Work out the finished part from the listing and answer in its coordinate system (mm). Face numbers are marked on the shaded views. A direction names the side the tool comes from. Round coordinates to 2 decimals unless told otherwise and drop trailing zeros. Order: outer loops, then holes, each group sorted by start corner. A loop starts at its lowest first (then second) coordinate and runs counter-clockwise, first axis right, second up. Notation, with made-up numbers: (-12, 83.5) - (31, 83.5) arc R27 cw to (31, 119.5) - close; hole circle Ø5 at (20, -11.75). An arc over 180 degrees is marked (long way). Put each result on its own line as item: value.
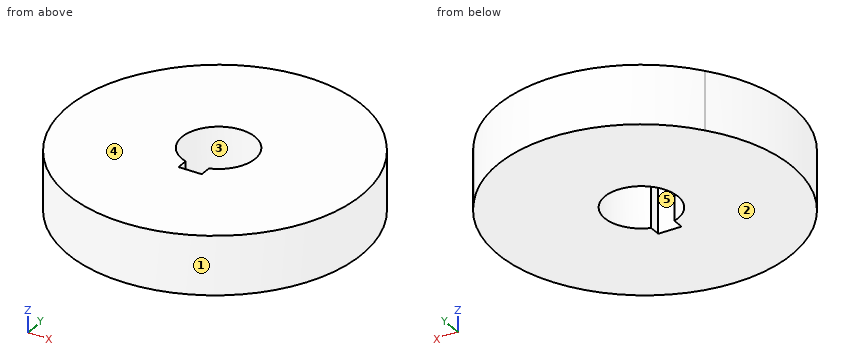
```python
from build123d import *

# Parameters (mm, degrees)
F1_DEPTH = 200
F3_DEPTH = 469.9


# Not quite as in the source:
# - a feature names something its author has since deleted; it is built from what else it names


with BuildPart() as f1:
    # F0 (on Top) → F1 (new body)
    with BuildSketch(Plane.XY):
        with BuildLine():
            ThreePointArc((-396.7193466419, 287.6), (-151.1746012819, -466.0968138995), (490, 0))
            ThreePointArc((490, 0), (466.0968138995, 151.1746012818), (396.7193466419, 287.6))
            ThreePointArc((396.7193466419, 287.6), (0, 482), (-396.7193466419, 287.6))
        make_face()
        with BuildLine():
            ThreePointArc((396.7193466419, 287.6), (466.0968138995, 151.1746012818), (490, 0))
            ThreePointArc((490, 0), (-151.1746012819, -466.0968138995), (-396.7193466419, 287.6))
            ThreePointArc((-396.7193466419, 287.6), (-162.5590477115, -494.9511090703), (502, -20))
            ThreePointArc((502, -20), (474.9511090703, 142.5590477115), (396.7193466419, 287.6))
        make_face()
        with BuildLine():
            ThreePointArc((-396.7193466419, 287.6), (0, 482), (396.7193466419, 287.6))
            ThreePointArc((396.7193466419, 287.6), (0, 490), (-396.7193466419, 287.6))
        make_face()
    extrude(amount=-F1_DEPTH)

    # F2 (on Top) → F3 (cut)
    with BuildSketch(Plane.XY):
        with BuildLine():
            ThreePointArc((40, -118.4271928233), (101.5504800579, -72.8868986856), (125, 0))
            ThreePointArc((125, 0), (-72.8868986856, 101.5504800579), (-40, -118.4271928233))
            Line((-40, -118.4271928233), (-40, 0))
            Line((-40, 0), (40, 0))
            Line((40, 0), (40, -118.4271928233))
        make_face()
        with BuildLine():
            Line((-40, 0), (-40, -118.4271928233))
            ThreePointArc((-40, -118.4271928233), (0, -125), (40, -118.4271928233))
            Line((40, -118.4271928233), (40, 0))
            Line((40, 0), (-40, 0))
        make_face()
        with BuildLine():
            ThreePointArc((40, -118.4271928233), (0, -125), (-40, -118.4271928233))
            Line((-40, -118.4271928233), (-40, -158))
            Line((-40, -158), (40, -158))
            Line((40, -158), (40, -118.4271928233))
        make_face()
    extrude(amount=-F3_DEPTH, mode=Mode.SUBTRACT)


solid = f1.part
```
1) For a pull along X with two mould halves and no side action, classify the marked faces 1, 2 and 3 as pulls with the +X half, pulls with the -X half, needs draft (parallel to the pull), parting line crosses it, or undercut.
Findings below:
face 1: parting line crosses it
face 2: needs draft
face 3: undercut
2) A cutting plane is placed at B-B on y = -20. Write down the section's boundary in (x, z).
Findings below:
outline: (-502, -200) - (-123.39, -200) - (-123.39, 0) - (-502, 0) - close; (123.39, -200) - (502, -200) - (502, 0) - (123.39, 0) - close
3) Given pin 1 Ø6 at (x, z) = (338.5, -51) entering from +Y; pin 2 Ø12 at (y, z) = (-134, -103) entering from +X; pin 3 Ø12 at (y, z) = (-197.5, -139) entering from -X, each flat-ended and moving along its own axis, determine where each tip first touches the part or whether it passes through.
Findings below:
pin 1: stops at y = 357.13
pin 2: stops at x = 490.24
pin 3: stops at x = -471.8
4) Straight lines are drawn through the part: L1, parallel to Y at x = 0, z = -56.5; L2, parallel to X at y = -153.5, z = -72; L3, parallel to X at y = -97, z = -34. For each, find the intervals that lie inside material, in ascending order. Write a range as from..to.
Findings below:
L1: y = -522..-158, 125..490
L2: x = -483.92..-40, 40..483.92
L3: x = -496.06..-78.84, 78.84..496.06
5) A cutting plane is placed at D-D on y = 342. Write down the section's boundary in (x, z).
Findings below:
outline: (-350.91, -200) - (350.91, -200) - (350.91, 0) - (-350.91, 0) - close
6) For the marked faces 4 and 5, determine the directions among +Z, -Z, +X, -X, +Y, -Y from which every point of the face is accessible in a straight line to the end or side of a thin tool.
Findings below:
face 4: +Z, +X, -X, +Y, -Y
face 5: +Z, -Z
7) A cutting plane is placed at C-C on z = -64. Write down the section's boundary in (x, y), then the cut area to 3 significant figures.
Findings below:
outline: (-396.72, 287.6) arc R502 ccw (long way) to (396.72, 287.6) arc R490 ccw to start; hole (-40, -158) - (40, -158) - (40, -118.43) arc R125 ccw (long way) to (-40, -118.43) - close
area: 745,000 mm2
8) A cutting plane is placed at A-A on x = 0. Write down the section's boundary in (y, z), then the cut area to 3 significant figures.
Findings below:
outline: (-522, -200) - (-158, -200) - (-158, 0) - (-522, 0) - close; (125, -200) - (490, -200) - (490, 0) - (125, 0) - close
area: 146,000 mm2
